from build123d import *

# Parameters (mm, degrees)
F0_R     = 2.5
F1_DEPTH = 152.4


with BuildPart() as f1:
    # F0 (on Top) → F1 (new body)
    with BuildSketch(Plane.XY):
        with BuildLine():
            ThreePointArc((-10.36, 12.5), (-11.873209, 11.873209), (-12.5, 10.36))
            Line((-12.5, 10.36), (-12.5, 4.32))
            ThreePointArc((-12.5, 4.32), (-11.43, 3.25), (-10.36, 4.32))
            Line((-10.36, 4.32), (-10.36, 6.263583))
            ThreePointArc((-10.36, 6.263583), (-9.699471, 7.252134), (-8.533396, 7.020187))
            Line((-8.533396, 7.020187), (-4.363396, 2.850187))
            ThreePointArc((-4.363396, 2.850187), (-4.131449, 2.503054), (-4.05, 2.093583))
            Line((-4.05, 2.093583), (-4.05, 0))
            Line((-4.05, 0), (-4.05, -2.093583))
            ThreePointArc((-4.05, -2.093583), (-4.131449, -2.503054), (-4.363396, -2.850187))
            Line((-4.363396, -2.850187), (-8.533396, -7.020187))
            ThreePointArc((-8.533396, -7.020187), (-9.699471, -7.252134), (-10.36, -6.263583))
            Line((-10.36, -6.263583), (-10.36, -4.32))
            ThreePointArc((-10.36, -4.32), (-11.43, -3.25), (-12.5, -4.32))
            Line((-12.5, -4.32), (-12.5, -12.5))
            Line((-12.5, -12.5), (-12.5, -20.68))
            ThreePointArc((-12.5, -20.68), (-11.43, -21.75), (-10.36, -20.68))
            Line((-10.36, -20.68), (-10.36, -18.736417))
            ThreePointArc((-10.36, -18.736417), (-9.699471, -17.747866), (-8.533396, -17.979813))
            Line((-8.533396, -17.979813), (-4.363396, -22.149813))
            ThreePointArc((-4.363396, -22.149813), (-4.131449, -22.496946), (-4.05, -22.906417))
            Line((-4.05, -22.906417), (-4.05, -25))
            Line((-4.05, -25), (-4.05, -27.093583))
            ThreePointArc((-4.05, -27.093583), (-4.131449, -27.503054), (-4.363396, -27.850187))
            Line((-4.363396, -27.850187), (-8.533396, -32.020187))
            ThreePointArc((-8.533396, -32.020187), (-9.699471, -32.252134), (-10.36, -31.263583))
            Line((-10.36, -31.263583), (-10.36, -29.32))
            ThreePointArc((-10.36, -29.32), (-11.43, -28.25), (-12.5, -29.32))
            Line((-12.5, -29.32), (-12.5, -35.36))
            ThreePointArc((-12.5, -35.36), (-11.873209, -36.873209), (-10.36, -37.5))
            Line((-10.36, -37.5), (-4.32, -37.5))
            ThreePointArc((-4.32, -37.5), (-3.25, -36.43), (-4.32, -35.36))
            Line((-4.32, -35.36), (-6.263583, -35.36))
            ThreePointArc((-6.263583, -35.36), (-7.252134, -34.699471), (-7.020187, -33.533396))
            Line((-7.020187, -33.533396), (-3.310187, -29.823396))
            ThreePointArc((-3.310187, -29.823396), (-2.963054, -29.591449), (-2.553583, -29.51))
            Line((-2.553583, -29.51), (0, -29.51))
            Line((0, -29.51), (2.553583, -29.51))
            ThreePointArc((2.553583, -29.51), (2.963054, -29.591449), (3.310187, -29.823396))
            Line((3.310187, -29.823396), (7.020187, -33.533396))
            ThreePointArc((7.020187, -33.533396), (7.252134, -34.699471), (6.263583, -35.36))
            Line((6.263583, -35.36), (4.32, -35.36))
            ThreePointArc((4.32, -35.36), (3.25, -36.43), (4.32, -37.5))
            Line((4.32, -37.5), (10.36, -37.5))
            ThreePointArc((10.36, -37.5), (11.873209, -36.873209), (12.5, -35.36))
            Line((12.5, -35.36), (12.5, -29.32))
            ThreePointArc((12.5, -29.32), (11.43, -28.25), (10.36, -29.32))
            Line((10.36, -29.32), (10.36, -31.263583))
            ThreePointArc((10.36, -31.263583), (9.699471, -32.252134), (8.533396, -32.020187))
            Line((8.533396, -32.020187), (4.363396, -27.850187))
            ThreePointArc((4.363396, -27.850187), (4.131449, -27.503054), (4.05, -27.093583))
            Line((4.05, -27.093583), (4.05, -25))
            Line((4.05, -25), (4.05, -22.906417))
            ThreePointArc((4.05, -22.906417), (4.131449, -22.496946), (4.363396, -22.149813))
            Line((4.363396, -22.149813), (8.533396, -17.979813))
            ThreePointArc((8.533396, -17.979813), (9.699471, -17.747866), (10.36, -18.736417))
            Line((10.36, -18.736417), (10.36, -20.68))
            ThreePointArc((10.36, -20.68), (11.43, -21.75), (12.5, -20.68))
            Line((12.5, -20.68), (12.5, -12.5))
            Line((12.5, -12.5), (12.5, -4.32))
            ThreePointArc((12.5, -4.32), (11.43, -3.25), (10.36, -4.32))
            Line((10.36, -4.32), (10.36, -6.263583))
            ThreePointArc((10.36, -6.263583), (9.699471, -7.252134), (8.533396, -7.020187))
            Line((8.533396, -7.020187), (4.363396, -2.850187))
            ThreePointArc((4.363396, -2.850187), (4.131449, -2.503054), (4.05, -2.093583))
            Line((4.05, -2.093583), (4.05, 0))
            Line((4.05, 0), (4.05, 2.093583))
            ThreePointArc((4.05, 2.093583), (4.131449, 2.503054), (4.363396, 2.850187))
            Line((4.363396, 2.850187), (8.533396, 7.020187))
            ThreePointArc((8.533396, 7.020187), (9.699471, 7.252134), (10.36, 6.263583))
            Line((10.36, 6.263583), (10.36, 4.32))
            ThreePointArc((10.36, 4.32), (11.43, 3.25), (12.5, 4.32))
            Line((12.5, 4.32), (12.5, 10.36))
            ThreePointArc((12.5, 10.36), (11.873209, 11.873209), (10.36, 12.5))
            Line((10.36, 12.5), (4.32, 12.5))
            ThreePointArc((4.32, 12.5), (3.25, 11.43), (4.32, 10.36))
            Line((4.32, 10.36), (6.263583, 10.36))
            ThreePointArc((6.263583, 10.36), (7.252134, 9.699471), (7.020187, 8.533396))
            Line((7.020187, 8.533396), (3.310187, 4.823396))
            ThreePointArc((3.310187, 4.823396), (2.963054, 4.591449), (2.553583, 4.51))
            Line((2.553583, 4.51), (0, 4.51))
            Line((0, 4.51), (-2.553583, 4.51))
            ThreePointArc((-2.553583, 4.51), (-2.963054, 4.591449), (-3.310187, 4.823396))
            Line((-3.310187, 4.823396), (-7.020187, 8.533396))
            ThreePointArc((-7.020187, 8.533396), (-7.252134, 9.699471), (-6.263583, 10.36))
            Line((-6.263583, 10.36), (-4.32, 10.36))
            ThreePointArc((-4.32, 10.36), (-3.25, 11.43), (-4.32, 12.5))
            Line((-4.32, 12.5), (-10.36, 12.5))
        make_face()
        with Locations((0, -25)):
            Circle(F0_R, mode=Mode.SUBTRACT)
        with BuildLine():
            Line((-2.553583, -4.51), (0, -4.51))
            Line((0, -4.51), (2.553583, -4.51))
            ThreePointArc((2.553583, -4.51), (2.963054, -4.591449), (3.310187, -4.823396))
            Line((3.310187, -4.823396), (7.646979, -9.160187))
            ThreePointArc((7.646979, -9.160187), (7.994112, -9.392134), (8.403583, -9.473583))
            Line((8.403583, -9.473583), (9.29, -9.473583))
            ThreePointArc((9.29, -9.473583), (10.046604, -9.786979), (10.36, -10.543583))
            Line((10.36, -10.543583), (10.36, -12.5))
            Line((10.36, -12.5), (10.36, -14.456417))
            ThreePointArc((10.36, -14.456417), (10.046604, -15.213021), (9.29, -15.526417))
            Line((9.29, -15.526417), (8.403583, -15.526417))
            ThreePointArc((8.403583, -15.526417), (7.994112, -15.607866), (7.646979, -15.839813))
            Line((7.646979, -15.839813), (3.310187, -20.176604))
            ThreePointArc((3.310187, -20.176604), (2.963054, -20.408551), (2.553583, -20.49))
            Line((2.553583, -20.49), (0, -20.49))
            Line((0, -20.49), (-2.553583, -20.49))
            ThreePointArc((-2.553583, -20.49), (-2.963054, -20.408551), (-3.310187, -20.176604))
            Line((-3.310187, -20.176604), (-7.646979, -15.839813))
            ThreePointArc((-7.646979, -15.839813), (-7.994112, -15.607866), (-8.403583, -15.526417))
            Line((-8.403583, -15.526417), (-9.29, -15.526417))
            ThreePointArc((-9.29, -15.526417), (-10.046604, -15.213021), (-10.36, -14.456417))
            Line((-10.36, -14.456417), (-10.36, -12.5))
            Line((-10.36, -12.5), (-10.36, -10.543583))
            ThreePointArc((-10.36, -10.543583), (-10.046604, -9.786979), (-9.29, -9.473583))
            Line((-9.29, -9.473583), (-8.403583, -9.473583))
            ThreePointArc((-8.403583, -9.473583), (-7.994112, -9.392134), (-7.646979, -9.160187))
            Line((-7.646979, -9.160187), (-3.310187, -4.823396))
            ThreePointArc((-3.310187, -4.823396), (-2.963054, -4.591449), (-2.553583, -4.51))
        make_face(mode=Mode.SUBTRACT)
        Circle(F0_R, mode=Mode.SUBTRACT)
    extrude(amount=F1_DEPTH)


solid = f1.part
Source: CAD feature listing. Evaluate the final solid. Frame: model axes, mm. A direction names the side the tool comes from. Coordinates: 2 decimals unless noted, no trailing zeros. Loops run counter-clockwise (first coordinate to the right, second up) from the corner with the lowest first, then second, coordinate; pieces in that order, holes last. Notation, with made-up numbers: (58, 64) - (110, 64) arc R20 ccw to (110, 84) - close; hole circle Ø10 at (-29.5, 43.5). An arc over 180 degrees is marked (long way). Return JSON: item names as keys, results as strings.
Q1. Mould query, pull axis Y, two halves, no side actions, for faces 1 (the flat face through (-5.509, -7.022, 75.133)), 2 (the flat face through (-12.5, -12, 75)), 3 (the flat face through (-7, 12.5, 75)), 4 (the flat face through (0, -20.49, 75)). Classes: released by +Y, released by -Y, zero draft, split by the parting line, or undercut.
Results:
{"face 1": "undercut", "face 2": "zero draft", "face 3": "released by +Y", "face 4": "undercut"}
Q2. Section A-A, the plane x = 0. Return loops of the section in (y, z).
Results:
{"outline": "(-29.51, 0) - (-27.5, 0) - (-27.5, 152.4) - (-29.51, 152.4) - close; (-22.5, 0) - (-20.49, 0) - (-20.49, 152.4) - (-22.5, 152.4) - close; (-4.51, 0) - (-2.5, 0) - (-2.5, 152.4) - (-4.51, 152.4) - close; (2.5, 0) - (4.51, 0) - (4.51, 152.4) - (2.5, 152.4) - close"}
Q3. Access query for faces 5 (the flat face through (12.5, 7, 75)), 6 (the flat face through (-4.05, 0, 75)), 7 (the flat face through (6.419, -20.094, 75.133)). Directions: +Z, -Z, +X, -X, +Y, -Y. A direction counts if a zero-diameter tool reaches every point of the face in a straight line with its end or side. Return the directions, or none.
Results:
{"face 5": "+Z, -Z, +X, +Y, -Y", "face 6": "+Z, -Z, -X", "face 7": "+Z, -Z"}
Q4. Section B-B, the plane y = 0. Return loops of the section in (x, z), plus the area to 3 significant figures.
Results:
{"outline": "(-4.05, 0) - (-2.5, 0) - (-2.5, 152.4) - (-4.05, 152.4) - close; (2.5, 0) - (4.05, 0) - (4.05, 152.4) - (2.5, 152.4) - close", "area": "472 mm2"}
Q5. Contact query for flat-ended pins moving along their axis: P1, Ø4.5, axis at y = -25.5, z = 73, coming from the -X side (3 decimals); P2, Ø1.3, axis at y = 0, z = 84.5, coming from the -X side; P3, Ø6, axis at x = 0.5, z = 16.5, coming from the -Y side. Output: stop coordinate, or through.
Results:
{"P1": "x = -4.275", "P2": "x = -4.05", "P3": "y = -37.12"}
Q6. Material intervals for line 1 along Y through (x, z) = (0, 57); line 2 along Y through (x, z) = (9.25, 24); line 3 along Y through (x, z) = (-4.75, 72.5), sorted ascending.
Results:
{"line 1": "-29.51 to -27.5, -22.5 to -20.49, -4.51 to -2.5, 2.5 to 4.51", "line 2": "-37.5 to -32.33, -17.67 to -15.53, -9.47 to -7.33, 7.33 to 12.5", "line 3": "-37.5 to -35.36, -31.26 to -28.24, -21.76 to -18.74, -6.26 to -3.24, 3.24 to 6.26, 10.36 to 12.5"}
Q7. Section C-C, the plane z = 105. Give the number of separate pieces and of enclosed holes in the cut face, plus the area to 3 significant figures.
Results:
{"separate pieces": "1", "enclosed holes": "3", "area": "476 mm2"}
